from build123d import *

# Parameters (mm, degrees)
F2_W = 15.708493
F2_H = 2.5
F4_R = 2.5


with BuildPart() as f1:
    # F0 (on Right) → F1 (revolve)
    with BuildSketch(Plane.YZ):
        with BuildLine():
            Line((-45, 4), (-45, 0))
            Line((-45, 0), (-45, -4))
            Line((-45, -4), (-26.497386, -4))
            ThreePointArc((-26.497386, -4), (-20.409772, -6.066467), (-16.838128, -11.41181))
            Line((-16.838128, -11.41181), (-11.992994, -29.494095))
            ThreePointArc((-11.992994, -29.494095), (-10.207172, -32.166767), (-7.163365, -33.2))
            Line((-7.163365, -33.2), (-4, -33.2))
            Line((-4, -33.2), (-4, 33.2))
            Line((-4, 33.2), (-7.163365, 33.2))
            ThreePointArc((-7.163365, 33.2), (-10.207172, 32.166767), (-11.992994, 29.494095))
            Line((-11.992994, 29.494095), (-16.838128, 11.41181))
            ThreePointArc((-16.838128, 11.41181), (-20.409772, 6.066467), (-26.497386, 4))
            Line((-26.497386, 4), (-45, 4))
        make_face()
    revolve(axis=Axis((0, 0, 0.106538), (0, 0, -1)))

    # F2 (on Right) → F3 (revolve)
    with BuildSketch(Plane.YZ):
        with Locations((48.145753, 1.25)):
            Rectangle(F2_W, F2_H)
    revolve(axis=Axis((0, 48.145753, 0), (0, 1, 0)))

    # F4
    f4_edges = [f1.edges().sort_by_distance(p)[0] for p in [
        (0, 56, -2.5),
    ]]
    fillet(f4_edges, radius=F4_R)


solid = f1.part
CAD build for the part. Positions are in the model's coordinates, mm. A direction names the side the tool comes from. Coordinates: 2 decimals unless noted, no trailing zeros. Write each loop counter-clockwise with the first axis right and the second up, starting at its lowest first coordinate (ties: lowest second). Pieces come first, ordered by that corner, then holes. Notation, with made-up numbers: M 77,89 L 96,89 A6 cw 96,93 Z; hole C -34,52 d6. An arc over 180 degrees is marked long. Return JSON: item names as keys, results as strings.
Item 1: Slice it at A-A, the plane y = 0. Write the cut outline in (x, z), and give its area (3 significant figures).
Findings below:
{"outline": "M -45,-4 L -26.5,-4 A10 cw -16.84,-11.41 L -11.99,-29.49 A5 ccw -7.16,-33.2 L -4,-33.2 L -4,33.2 L -7.16,33.2 A5 ccw -11.99,29.49 L -16.84,11.41 A10 cw -26.5,4 L -45,4 Z; M 4,-33.2 L 7.16,-33.2 A5 ccw 11.99,-29.49 L 16.84,-11.41 A10 cw 26.5,-4 L 45,-4 L 45,4 L 26.5,4 A10 cw 16.84,11.41 L 11.99,29.49 A5 ccw 7.16,33.2 L 4,33.2 Z", "area": "1,960 mm2"}
Item 2: Drop flat-ended pins along their axis: pin 1 Ø10 at (x, y) = (-11, 31.5) entering from +Z; pin 2 Ø5 at (y, z) = (8, 15) entering from +X; pin 3 Ø8 at (x, z) = (11.5, -18) entering from +Y. Give the stop position or say it passes through.
Findings below:
{"pin 1": "stops at z = 4", "pin 2": "stops at x = 15.13", "pin 3": "stops at y = 13.38"}
Item 3: Probe line 1 (X direction, y = 0, z = 3); line 2 (Z direction, x = -30.5, y = -9); line 3 (X direction, y = 0, z = 10). List the from-to ranges inside material, lowest first. Write a range as from..to.
Findings below:
{"line 1": "x = -45..-4, 4..45", "line 2": "z = -4..4", "line 3": "x = -17.33..-4, 4..17.33"}
Item 4: Which spindle directions (+Z, -Z, +X, -X, +Y, -Y) get a long thin tool onto all of the face, cutting with end or side? Do faces 4 (the flat face through (3, 3, 33.2)), 5 (the cylindrical face through (-2.44, 49.28, -0.54)), 6 (the flat face through (19, 19, 4)). Say none if no direction does.
Findings below:
{"face 4": "+Z, +X, -X, +Y, -Y", "face 5": "+Y", "face 6": "+Z"}
Item 5: Slice it at B-B, the plane x = 0. Write the cut outline in (y, z), and give its area (3 significant figures).
Findings below:
{"outline": "M -45,-4 L -26.5,-4 A10 cw -16.84,-11.41 L -11.99,-29.49 A5 ccw -7.16,-33.2 L -4,-33.2 L -4,33.2 L -7.16,33.2 A5 ccw -11.99,29.49 L -16.84,11.41 A10 cw -26.5,4 L -45,4 Z; M 4,-33.2 L 7.16,-33.2 A5 ccw 11.99,-29.49 L 16.84,-11.41 A10 cw 26.5,-4 L 45,-4 L 45,-2.5 L 53.5,-2.5 A2.5 ccw 53.5,2.5 L 45,2.5 L 45,4 L 26.5,4 A10 cw 16.84,11.41 L 11.99,29.49 A5 ccw 7.16,33.2 L 4,33.2 Z", "area": "2,020 mm2"}
Item 6: Two-plate mould, pull along X, no slides. Class faces 1 (the flat face through (19, -19, -4)), 2 (the cylindrical face through (3.905, 0.867, 0.465)), 3 (the cylindrical face through (17.235, -41.569, -0.056)): +X half, -X half, draft (parallel to the pull), parting line (faces both ways), or undercut.
Findings below:
{"face 1": "draft", "face 2": "undercut", "face 3": "parting line"}
Item 7: Slice it at C-C, the plane z = 0. Write the cut outline in (x, y), and give its area (3 significant figures).
Findings below:
{"outline": "M -2.5,44.93 A45 ccw long 2.5,44.93 L 2.5,53.5 A2.5 ccw -2.5,53.5 Z; hole C 0,0 d8", "area": "6,360 mm2"}
Item 8: Slice it at D-D, the plane y = 48. Write the cut outline in (x, z).
Findings below:
{"outline": "C 0,0 d5"}
